The listing builds one solid part. Answer for the finished solid, in the listing's coordinates (mm). A direction names the side the tool comes from. Coordinates: 2 decimals unless noted, no trailing zeros. Order: outer loops, then holes, each group sorted by start corner. A loop starts at its lowest first (then second) coordinate and runs counter-clockwise, first axis right, second up. Notation, with made-up numbers: (63, 8) -> (74, 8) arc R24 cw to (74, 31) -> close; hole circle Ø9 at (46, 61). An arc over 180 degrees is marked (long way). Write each question's results on one line, items separated by ' | '. Start each with the question number.
(1) The part is cut by section D-D, the plane z = 70. Give the vertices of the cut face in (x, y).
(2) Straight lines are drawn through the part: L1, parallel to Z at x = -2, y = -26; L2, parallel to Z at x = 38.5, y = -31; L3, parallel to X at y = -39, z = 19. For each, find the intervals that lie inside material, in ascending order.
(3) Given pin 1 (8 mm diameter, centred on x = 49, y = -40.5, fed in from -Z); pin 2 (5 mm diameter, centred on x = 14.5, y = -44, fed in from +Z); pin 3 (5 mm diameter, centred on y = -27, z = 72, fed in from +X), each flat-ended and moving along its own axis, determine where each tip first touches the part or whether it passes through.
(4) Determine the mould class of faces 1 (the face through (26.9, 0, 4.8)), 2 (the face through (-2.535, -25.133, 66.095)), 3 (the face through (26.9, -50, 4.8)), 4 (the face through (85, -25, 2)) for opening direction Y: +Y half, -Y half, draft (parallel to the pull), parting line (faces both ways), or undercut.
(5) The part is cut by section B-B, the plane y = -26. Give the vertices of the cut face in (x, z), then the cut area to 3 significant figures.
(6) The part is cut by section A-A, the plane z = 25.72. Give the vertices of the cut face in (x, y), then the cut area to 3 significant figures.
(7) A tool of negligible diameter and unlimited length cuts with its end or side. For faces 5 (the face through (0, -25, 47)), 6 (the face through (-5, -25, 44)), from which of +Z, -Z, +X, -X, +Y, -Y can it reach the whole face along a straight path? Write none if from no direction.
(8) The part is cut by section C-C, the plane y = -40. Give the vertices of the cut face in (x, z).
```python
from build123d import *

# Parameters (mm, degrees)
SKETCH1_W           = 85
SKETCH1_H           = 50
BOSS_EXTRUDE1_DEPTH = 5
SKETCH2_W           = 90
SKETCH2_H           = 50
BOSS_EXTRUDE2_DEPTH = 5
SKETCH3_R           = 4
SKETCH3_R_2         = 5
CUT_EXTRUDE1_DEPTH  = 5


with BuildPart() as part:
    # Sketch1 → Boss-Extrude1 (new body)
    with BuildSketch(Plane.XY):
        with Locations((42.5, -25)):
            Rectangle(SKETCH1_W, SKETCH1_H)
    extrude(amount=BOSS_EXTRUDE1_DEPTH)

    # Sketch2 → Boss-Extrude2 (add)
    with BuildSketch(Plane.ZY):
        with Locations((45, -25)):
            Rectangle(SKETCH2_W, SKETCH2_H)
    extrude(amount=BOSS_EXTRUDE2_DEPTH)

    # Sketch3 → Cut-Extrude1 (cut)
    with BuildSketch(Plane.ZY.offset(5)):
        with Locations(Location((70, -26, 0), (0, 0, 270))):
            Circle(SKETCH3_R)
        with Locations(Location((25.72, -26, 0), (0, 0, 270))):
            Circle(SKETCH3_R_2)
    extrude(amount=-CUT_EXTRUDE1_DEPTH, mode=Mode.SUBTRACT)


solid = part.part
```
Established:
1) outline: (-5, -50) -> (0, -50) -> (0, -30) -> (-5, -30) -> close; (-5, -22) -> (0, -22) -> (0, 0) -> (-5, 0) -> close
2) L1: z = 0 to 20.72, 30.72 to 66, 74 to 90 | L2: z = 0 to 5 | L3: x = -5 to 0
3) pin 1: stops at z = 0 | pin 2: stops at z = 5 | pin 3: stops at x = 0
4) face 1: +Y half | face 2: undercut | face 3: -Y half | face 4: draft
5) outline: (-5, 0) -> (85, 0) -> (85, 5) -> (0, 5) -> (0, 20.72) -> (-5, 20.72) -> close; (-5, 30.72) -> (0, 30.72) -> (0, 66) -> (-5, 66) -> close; (-5, 74) -> (0, 74) -> (0, 90) -> (-5, 90) -> close | area: 785 mm^2
6) outline: (-5, -50) -> (0, -50) -> (0, -31) -> (-5, -31) -> close; (-5, -21) -> (0, -21) -> (0, 0) -> (-5, 0) -> close | area: 200 mm^2
7) face 5: +Z, +X, +Y, -Y | face 6: +Z, -Z, -X, +Y, -Y
8) outline: (-5, 0) -> (85, 0) -> (85, 5) -> (0, 5) -> (0, 90) -> (-5, 90) -> close
